For this review, take the finished solid that the model builds, in its own axes (mm). A direction names the side the tool comes from. Coordinates: 2 decimals unless noted, no trailing zeros. Write each loop counter-clockwise with the first axis right and the second up, starting at its lowest first coordinate (ties: lowest second). Pieces come first, ordered by that corner, then holes. Notation, with made-up numbers: M 64,-14.5 L 73,-14.5 A24 ccw 73,-4.5 Z; hole C 19,-32 d6. An arc over 180 degrees is marked long. Return JSON: item names as keys, results as strings.
```python
from build123d import *

# Parameters (mm, degrees)
BOSS_EXTRUDE1_DEPTH = 17.5
SKETCH3_R           = 2.25
CUT_EXTRUDE1_DEPTH  = 56.7
CHAMFER1_SIZE       = 0.4
CHAMFER2_SIZE       = 0.4
CHAMFER3_SIZE       = 0.4


with BuildPart() as part:
    # Sketch1 → Revolve1 (revolve)
    with BuildSketch(Plane.XY):
        Polygon((0, 0), (-19, 0), (-19, 50.7), (-28.5, 50.7), (-28.5, 55.7), (-12.5, 55.7), (-12.5, 58.7), (-5, 58.7), (-5, 60.2), (0, 60.2), align=None)
    revolve(axis=Axis((0, 60.2, 0), (0, -1, 0)))

    # Sketch2 → Boss-Extrude1 (add)
    with BuildSketch(Plane(origin=(0, 60.2, 0), x_dir=(1, 0, 0), z_dir=(0, 1, 0))):
        with BuildLine():
            Line((-1.936491673, 3.5), (1.936491673, 3.5))
            ThreePointArc((1.936491673, 3.5), (0, -4), (-1.936491673, 3.5))
        make_face()
    extrude(amount=BOSS_EXTRUDE1_DEPTH)

    # Sketch3 → Cut-Extrude1 (cut, through all)
    with BuildSketch(Plane(origin=(0, 55.7, 0), x_dir=(1, 0, 0), z_dir=(0, 1, 0))):
        with Locations((-25, 0)):
            Circle(SKETCH3_R)
        with Locations((0, 25)):
            Circle(SKETCH3_R)
        with Locations((25, 0)):
            Circle(SKETCH3_R)
        with Locations((0, -25)):
            Circle(SKETCH3_R)
    extrude(amount=-CUT_EXTRUDE1_DEPTH, mode=Mode.SUBTRACT)

    # Chamfer1
    chamfer1_edges = [part.edges().sort_by_distance(p)[0] for p in [
        (28.5, 55.7, 0),
        (28.5, 50.7, 0),
        (12.5, 58.7, 0),
    ]]
    chamfer(chamfer1_edges, length=CHAMFER1_SIZE)

    # Chamfer2
    chamfer2_edges = [part.edges().sort_by_distance(p)[0] for p in [
        (0, 77.7, 4),
    ]]
    chamfer(chamfer2_edges, length=CHAMFER2_SIZE)

    # Chamfer3
    chamfer3_edges = [part.edges().sort_by_distance(p)[0] for p in [
        (5, 60.2, 0),
    ]]
    chamfer(chamfer3_edges, length=CHAMFER3_SIZE)


solid = part.part
```
1. Clearance check with flat-ended pins moving along their axes: pin 1 Ø1 at (x, z) = (3.5, 14) entering from +Y; pin 2 Ø12 at (y, z) = (22.5, -2) entering from -X; pin 3 Ø1.9 at (x, y) = (-1, 73) entering from -Z. State where each tip first meets the part, or that it passes through.
Checks:
{"pin 1": "y = 55.7", "pin 2": "x = -19", "pin 3": "z = -3.5"}
2. We need section A-A (y = 52.5). State the section outline as (x, z) points, plus the area to 3 significant figures.
Checks:
{"outline": "C 0,0 d57; hole C -25,0 d4.5; hole C 0,-25 d4.5; hole C 0,25 d4.5; hole C 25,0 d4.5", "area": "2,490 mm2"}
3. Wall thickness on L1, parallel to Z at x = 0, y = 54.6; L2, parallel to Y at x = -19, z = -2.5; L3, parallel to Y at x = 11.5, z = 6: over which ranges is each line inside the solid? List them lowest first. Write a range as from..to.
Checks:
{"L1": "-28.5..-27.25, -22.75..22.75, 27.25..28.5", "L2": "50.7..55.7", "L3": "0..55.7"}
4. Draft analysis for pull direction X (two halves, no side actions). For faces 1 (the face through (-22.854, 53.235, -0.676)), 2 (the face through (5.9, 50.7, 18.3)), 3 (the face through (-8.767, 25.705, 16.856)), state which applies: +X half, -X half, draft (parallel to the pull), parting line (faces both ways), or undercut.
Checks:
{"face 1": "undercut", "face 2": "draft", "face 3": "parting line"}
5. We need section C-C (y = 62.5). State the section outline as (x, z) points.
Checks:
{"outline": "M -1.94,-3.5 L 1.94,-3.5 A4 ccw long Z"}
6. For faces 4 (the face through (-0.488, 53.235, -22.804)), 5 (the face through (-5.2, 58.7, -0.2)), list the 3-axis set-ups (+Z, -Z, +X, -X, +Y, -Y) from which the entire face can be reached by the end or side of a thin tool; tool diameter is ignored.
Checks:
{"face 4": "+Y, -Y", "face 5": "+Y"}
7. We need section D-D (y = 26.5). State the section outline as (x, z) points, plus the area to 3 significant figures.
Checks:
{"outline": "C 0,0 d38", "area": "1,130 mm2"}
8. We need section B-B (z = 0). Give the number of separate pieces and of enclosed holes in the cut face, plus the area to 3 significant figures.
Checks:
{"separate pieces": "3", "enclosed holes": "0", "area": "2,400 mm2"}
